Source: three-view drawing plus pictorial views. Frame: mm from the lowest corner of the part. Give positions to 0.01 mm unless a question says otherwise; leave off trailing zeros. Loops run counter-clockwise (first coordinate to the right, second up) from the corner with the lowest first, then second, coordinate; pieces in that order, holes last.
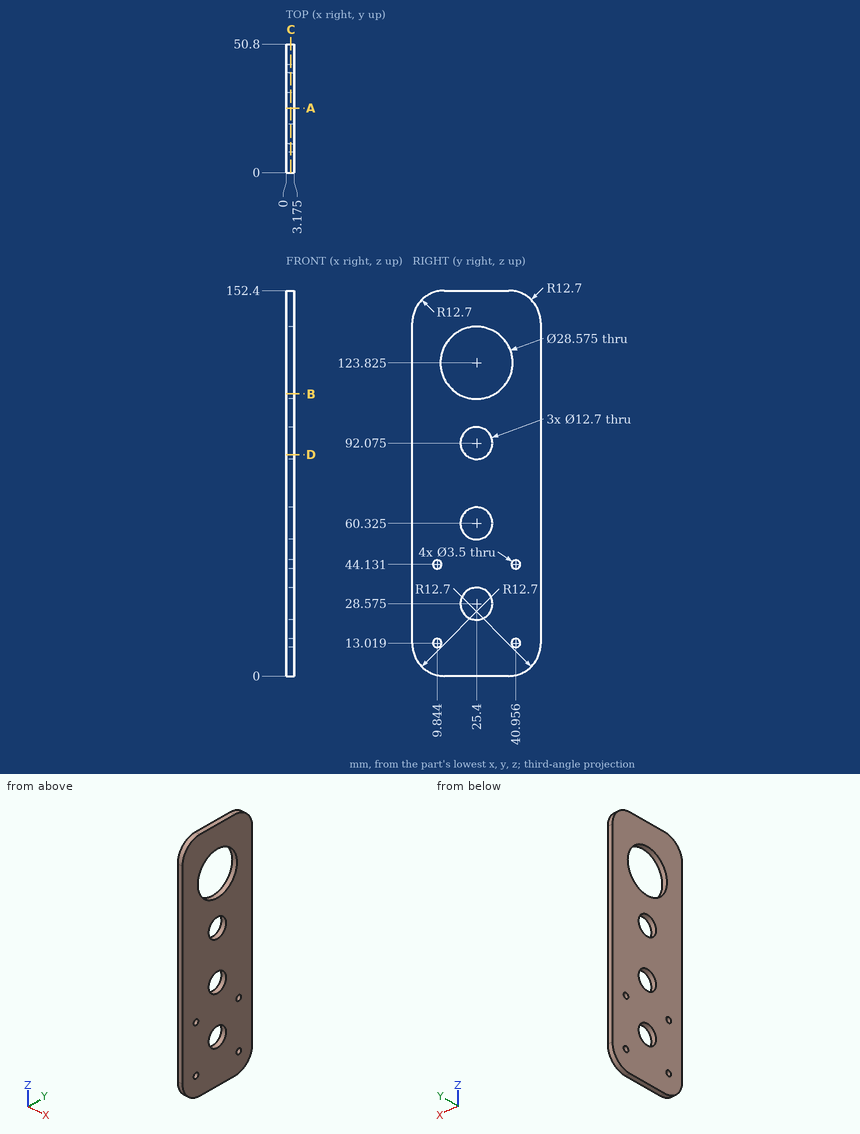
(1) Cut plane C-C (x = 1.8). Count the separate pieces of the cut face and the enclosed holes in it, and give its area (3 significant figures).
Values follow:
separate pieces: 1
enclosed holes: 8
area: 6,540 mm2
(2) Cut plane D-D (z = 87.5). Return the cut outline in (x, y) (1 decimal), and give its area (3 significant figures).
Values follow:
outline: (0, 0) - (3.2, 0) - (3.2, 21) - (0, 21) - close; (0, 29.8) - (3.2, 29.8) - (3.2, 50.8) - (0, 50.8) - close
area: 133 mm2
(3) Cut plane B-B (z = 111.5). Return the cut outline in (x, y) (1 decimal).
Values follow:
outline: (0, 0) - (3.2, 0) - (3.2, 18.2) - (0, 18.2) - close; (0, 32.6) - (3.2, 32.6) - (3.2, 50.8) - (0, 50.8) - close
(4) Ray query, probe 1 along Z at (x, y) = (0.9, 25.4) (1 decimal); probe 2 along Y at (x, z) = (1.95, 92); probe 3 along Y at (x, z) = (1.25, 45.5) (1 decimal). Return the intervals inside material, ascending.
Values follow:
probe 1: z = 0 to 22.2, 34.9 to 54, 66.7 to 85.7, 98.4 to 109.5, 138.1 to 152.4
probe 2: y = 0 to 19.05, 31.75 to 50.8
probe 3: y = 0 to 8.8, 10.9 to 39.9, 42 to 50.8
(5) Cut plane A-A (y = 25.4). Return the cut outline in (x, z) (1 decimal), and give its area (3 significant figures).
Values follow:
outline: (0, 0) - (3.2, 0) - (3.2, 22.2) - (0, 22.2) - close; (0, 34.9) - (3.2, 34.9) - (3.2, 54) - (0, 54) - close; (0, 66.7) - (3.2, 66.7) - (3.2, 85.7) - (0, 85.7) - close; (0, 98.4) - (3.2, 98.4) - (3.2, 109.5) - (0, 109.5) - close; (0, 138.1) - (3.2, 138.1) - (3.2, 152.4) - (0, 152.4) - close
area: 272 mm2
